Autodesk Inventor part; units mm, degrees
ref_plane "YZ Plane" through (0, 0, 0) normal (1, 0, 0) x (0, 1, 0)
ref_plane "XZ Plane" through (0, 0, 0) normal (0, 1, 0) x (-1, 0, 0)
ref_plane "XY Plane" through (0, 0, 0) normal (0, 0, 1) x (1, 0, 0)
sketch "Sketch1" plane through (0, 0, 0) normal (0, 0, 1) x (1, 0, 0)
  line L0 (0, 0) -> (38.1, 0)
  line L1 (38.1, 0) -> (38.1, 253.0348)
  arc A0 (38.1, 507.0348) -> (38.1, 253.0348) centre (666.75, 380.0348) ccw
  line L2 (38.1, 507.0348) -> (38.1, 608.6348)
  line L3 (38.1, 608.6348) -> (0, 608.6348)
  line L4 (0, 608.6348) -> (0, 0)
  circle A1 centre (31.75, 151.4348) radius 3.3655
  circle A2 centre (31.75, 34.671) radius 3.3655
  circle A3 centre (12.7, 12.7) radius 3.3655
  circle A4 centre (12.7, 342.9) radius 3.3655
  circle A5 centre (12.7, 595.9348) radius 3.3655
  circle A6 centre (31.75, 12.7) radius 3.3655
  circle A7 centre (31.75, 253.0348) radius 3.3655
  circle A8 centre (31.75, 507.0348) radius 3.3655
  circle A9 centre (31.75, 595.9348) radius 3.3655
  line L5 (0, 557.8348) -> (0, 608.6348)
  line L6 (0, 50.8) -> (0, 0)
  line L7 (12.7, 342.9) -> (0, 304.3174) construction
  line L8 (0, 317.5) -> (0, 368.3)
  line L9 (0, 129.921) -> (12.7, 129.921) construction
  circle A10 centre (12.7, 129.921) radius 3.3655
  circle A11 centre (12.7, 174.371) radius 3.3655
  line L10 (9.3413, 197.482) -> (9.3413, 204.213)
  line L11 (16.0611, 204.488) -> (16.0611, 197.3435)
  arc A12 (16.0611, 204.488) -> (9.3413, 204.213) centre (12.6956, 204.488) ccw
  arc A13 (9.3413, 197.482) -> (16.0611, 197.3435) centre (12.6974, 197.231) ccw
  circle A14 centre (12.7, 217.188) radius 3.3655
  dimension "d0" = 38.1
  dimension "d2" = 101.6
  dimension "d4" = 457.2
  dimension "d5" = 101.6
  dimension "d6" = 666.75
  dimension "d7" = 641.35
  dimension "d9" = 116.7638
  dimension "d10" = 6.35
  dimension "d11" = 6.35
  dimension "d13" = 12.7
  dimension "d14" = 12.7
  dimension "d16" = 12.7
  dimension "d17" = 342.9
  dimension "d19" = 12.7
  dimension "d20" = 12.7
  dimension "d22" = 6.35
  dimension "d24" = 6.35
  dimension "d25" = 6.731
  dimension "d26" = 6.35
  dimension "hole" = 6.731
  dimension "d28" = 6.35
  dimension "d45" = 12.7
  dimension "d47" = 12.7
  dimension "d54" = 6.731
  dimension "d55" = 3.3655
  dimension "d56" = 3.3655
  dimension "d58" = 6.731
  dimension "d59" = 12.7
  dimension "d68" = 18.22
  dimension "d69" = 90
  dimension "d70" = 90
  dimension "d71" = 22.0389
  dimension "d72" = 28.7587
  dimension "d73" = 478.7138
  dimension "d74" = 6.35
  dimension "d75" = 6.35
  dimension "d76" = 595.9348
  dimension "d77" = 404.1468
  dimension "d78" = 411.2913
  dimension "d79" = 25.4
  dimension "d80" = 25.4
  dimension "d81" = 434.2638
  dimension "d82" = 50.8
  dimension "d83" = 240.3348
  dimension "d84" = 291.1348
  dimension "d85" = 557.8348
extrude "Plate4" add sketch "Sketch1" along normal blind 3.048
sketch "Sketch5" plane through (0, 0, 3.048) normal (0, 0, 1) x (1, 0, 0)
  line L0 (38.1, 0) -> (38.1, 253.0348)
  line L1 (0, 0) -> (38.1, 0)
  line L2 (38.1, 0) -> (38.1, 25.4)
  line L3 (38.1, 25.4) -> (0, 25.4)
  line L4 (0, 25.4) -> (0, 0)
  dimension "d96" = 25.4
extrude "Cut1" cut sketch "Sketch5" against normal blind 3.048
sketch "Sketch7" plane through (0, 25.4, 3.048) normal (-1, 0, 0) x (0, -1, 0)
  line L0 (-583.2348, 0) -> (0, 0)
  line L1 (0, 0) -> (0, 22.352)
  line L2 (0, 22.352) -> (-583.2348, 22.352)
  line L3 (-583.2348, 22.352) -> (-583.2348, 0)
edge flange "Flange3" height 25.4 angle 90 thickness 3.048 bend radius 3.048 thickness toward (-1, 0, 0) relief tear relief width 3.048 relief depth 1.524 edges at (0, 317.0174, 3.048) wall of the first edge with corners at (0, 608.6348, 3.048) (0, 25.4, 3.048) (0, 25.4, 25.4) (0, 608.6348, 25.4)
bend "Bend3"
corner "Corner3"
sketch "Sketch9" plane through (38.1, 25.4, 0) normal (0, -1, 0) x (1, 0, 0)
  line L0 (0, 0) -> (-41.148, 0)
  line L1 (-41.148, 0) -> (-41.148, 25.4)
  line L2 (-41.148, 25.4) -> (0, 25.4)
  line L3 (0, 25.4) -> (0, 0)
  point P0 (-38.1, 0)
extrude "Extrusion2" cut sketch "Sketch9" against normal blind 513.3848
equation "\"d25\" = hole"
equation "\"d97\" = Thickness"
equation "\"d109\" = BendReliefWidth"
equation "\"d110\" = BendReliefDepth"
equation "\"d111\" = MinimumRemnant"
equation "\"d112\" = BendRadius"
equation "\"d115\" = BendRadius"
equation "\"d116\" = CornerReliefSize"
equation "\"d117\" = GapSize"
equation "\"d118\" = JacobiRadiusSize"
equation "\"BendRadius\" = Thickness"
equation "\"BendReliefWidth\" = Thickness"
equation "\"BendReliefDepth\" = 0.5 * Thickness"
equation "\"CornerReliefSize\" = 4 * Thickness"
equation "\"MinimumRemnant\" = 2 * Thickness"
equation "\"TransitionRadius\" = BendRadius"
equation "\"JacobiRadiusSize\" = BendRadius"
equation "\"GapSize\" = Thickness"
equation "\"d29\" = BendRadius"
equation "\"d32\" = BendRadius"
equation "\"d38\" = BendRadius"
equation "\"d60\" = BendRadius"
properties part number "Claw - Arm - Top (R) Top"
Verification items for the finished model (mm, model axes). A direction names the side the tool comes from. Coordinates: 2 decimals unless noted, no trailing zeros. Order: outer loops, then holes, each group sorted by start corner. A loop starts at its lowest first (then second) coordinate and runs counter-clockwise, first axis right, second up. Notation, with made-up numbers: (1.5, 83.5) -> (36.5, 83.5) arc R11 cw to (36.5, 100.5) -> close; hole circle Ø1 at (40, -16). An arc over 180 degrees is marked (long way). Put each result on its own line as item: value. Start each with the question number.
1. Mould release check, pull along Y, two halves, no side actions. Record for faces 3 (the flat face through (10, 608.635, 2)), 4 (the flat face through (-3.048, 573, 16)), 5 (the cylindrical face through (11.97, 599.22, 1.5)), 6 (the cylindrical face through (29.079, 597.983, 1.503)): released by +Y, released by -Y, zero draft, split by the parting line, or undercut.
2. Cross-section at B-B, the plane y = 563.5. Record the boundary of the cut face in (x, z).
3. Material ranges on L1, parallel to Y at x = 31.75, z = 1.6; L2, parallel to X at y = 567.5, z = 6.75; L3, parallel to Z at x = 27, y = 556.5, recorded low to high. Write a range as [from, to].
4. Access from +Z, -Z, +X, -X, +Y, -Y to the whole of each face (thin tool, end or side, straight path). Record for faces 1 (the flat face through (0, 573, 16)), 2 (the flat face through (-2, 573, 25.4)).
5. Cross-section at D-D, the plane z = 7.25. Record the boundary of the cut face in (x, y).
6. Cross-section at C-C, the plane x = 31. Record the boundary of the cut face in (y, z).
7. Cross-section at A-A, the plane x = 12.7. Record the boundary of the cut face in (y, z), then the cut area to 3 significant figures.
8. Go/stop test with flat-tipped pins: pin 1 Ø4 at (y, z) = (569.5, 16) entering from +X; pin 2 Ø1 at (x, y) = (23.5, 549) entering from +Z; pin 3 Ø1.5 at (x, y) = (20, 556.5) entering from -Z; pin 4 Ø1.5 at (y, z) = (559.5, 5.5) entering from +X. Record where each tip stops, or that it passes through.
Computed:
1. face 3: released by +Y
1. face 4: zero draft
1. face 5: undercut
1. face 6: undercut
2. outline: (-3.05, 6.1) arc R6.1 ccw to (3.05, 0) -> (38.1, 0) -> (38.1, 3.05) -> (3.05, 3.05) arc R3.05 cw to (0, 6.1) -> (0, 25.4) -> (-3.05, 25.4) -> close
3. L1: [538.78, 592.57], [599.3, 608.63]
3. L2: [-3.05, 0]
3. L3: [0, 3.05]
4. face 1: +Z, +X, +Y, -Y
4. face 2: +Z, +X, -X, +Y, -Y
5. outline: (-3.05, 538.78) -> (0, 538.78) -> (0, 608.63) -> (-3.05, 608.63) -> close
6. outline: (538.78, 0) -> (592.65, 0) -> (592.65, 3.05) -> (538.78, 3.05) -> close; (599.22, 0) -> (608.63, 0) -> (608.63, 3.05) -> (599.22, 3.05) -> close
7. outline: (538.78, 0) -> (592.57, 0) -> (592.57, 3.05) -> (538.78, 3.05) -> close; (599.3, 0) -> (608.63, 0) -> (608.63, 3.05) -> (599.3, 3.05) -> close
7. area: 192 mm2
8. pin 1: x = 0
8. pin 2: z = 3.05
8. pin 3: z = 0
8. pin 4: x = 0.31
